from build123d import *

# Parameters (mm, degrees)
SKETCH1_R           = 1.5
SKETCH1_R_2         = 4.925
SKETCH1_W           = 9.9
SKETCH1_H           = 6.4
SKETCH1_W_2         = 6.4
SKETCH1_H_2         = 9.4
BOSS_EXTRUDE1_DEPTH = 6.4
SKETCH2_R           = 1.5
SKETCH2_W           = 6.4
SKETCH2_H           = 9.9
CUT_EXTRUDE1_DEPTH  = 415.760486883


with BuildPart() as part:
    # Sketch1 → Boss-Extrude1 (new body)
    with BuildSketch(Plane(origin=(0, 0, 0), x_dir=(0, 0, -1), z_dir=(1, 0, 0))):
        Polygon((210.165001125, 41.275232149), (-37.634998875, 41.275232149), (-73.734998875, 5.175232149), (-73.734998875, -333.674767851), (-33.721689147, -333.674767851), (-18.721689147, -318.674767851), (175.325001125, -318.674767851), (190.325001125, -333.674767851), (246.265001125, -333.674767851), (246.265001125, 5.175232149), align=None)
        with Locations((6.365001125, 34.475232149)):
            Circle(SKETCH1_R, mode=Mode.SUBTRACT)
        with Locations((86.365001125, 34.475232149)):
            Circle(SKETCH1_R, mode=Mode.SUBTRACT)
        with Locations((166.365001125, 34.475232149)):
            Circle(SKETCH1_R, mode=Mode.SUBTRACT)
        with Locations((86.46500109, -259.124767851)):
            Circle(SKETCH1_R, mode=Mode.SUBTRACT)
        with Locations((166.465001125, -259.124767851)):
            Circle(SKETCH1_R, mode=Mode.SUBTRACT)
        with Locations((6.46500109, -259.124767851)):
            Circle(SKETCH1_R, mode=Mode.SUBTRACT)
        with Locations((239.465001125, -29.824767851)):
            Circle(SKETCH1_R, mode=Mode.SUBTRACT)
        with Locations((239.465001125, -136.224767851)):
            Circle(SKETCH1_R, mode=Mode.SUBTRACT)
        with Locations((239.465001125, -242.624767851)):
            Circle(SKETCH1_R, mode=Mode.SUBTRACT)
        with Locations((-66.934998875, -242.624767851)):
            Circle(SKETCH1_R, mode=Mode.SUBTRACT)
        with Locations((-66.934998875, -136.224767851)):
            Circle(SKETCH1_R, mode=Mode.SUBTRACT)
        with Locations((-66.934998875, -29.824767851)):
            Circle(SKETCH1_R, mode=Mode.SUBTRACT)
        with Locations((224.265001125, 13.800232149)):
            Circle(SKETCH1_R_2, mode=Mode.SUBTRACT)
        with Locations((-51.734998875, 13.800232149)):
            Circle(SKETCH1_R_2, mode=Mode.SUBTRACT)
        with Locations((193.115001125, -15.324767851)):
            Circle(SKETCH1_R, mode=Mode.SUBTRACT)
        with Locations((193.115001125, -34.074767851)):
            Circle(SKETCH1_R, mode=Mode.SUBTRACT)
        with Locations((151.365001054, 34.475232149)):
            Rectangle(SKETCH1_W, SKETCH1_H, mode=Mode.SUBTRACT)
        with Locations((181.365001197, 34.475232149)):
            Rectangle(SKETCH1_W, SKETCH1_H, mode=Mode.SUBTRACT)
        with Locations((71.365001054, 34.475232149)):
            Rectangle(SKETCH1_W, SKETCH1_H, mode=Mode.SUBTRACT)
        with Locations((101.365001197, 34.475232149)):
            Rectangle(SKETCH1_W, SKETCH1_H, mode=Mode.SUBTRACT)
        with Locations((21.465001197, -259.124767851)):
            Rectangle(SKETCH1_W, SKETCH1_H, mode=Mode.SUBTRACT)
        Polygon((157.825001125, 6.525232149), (189.675001125, -25.324767851), (189.675001125, -206.824767851), (-34.371689147, -206.824767851), (-34.371689147, -25.324767851), (-2.521689147, 6.525232149), align=None, mode=Mode.SUBTRACT)
        Polygon((-3.584998946, -255.924767851), (-3.584999089, -262.324767851), (-13.484999089, -262.324767851), (-13.484998946, -255.924767851), align=None, mode=Mode.SUBTRACT)
        with Locations((101.465001197, -259.124767851)):
            Rectangle(SKETCH1_W, SKETCH1_H, mode=Mode.SUBTRACT)
        with Locations((-8.634998946, 34.475232149)):
            Rectangle(SKETCH1_W, SKETCH1_H, mode=Mode.SUBTRACT)
        with Locations((21.365001197, 34.475232149)):
            Rectangle(SKETCH1_W, SKETCH1_H, mode=Mode.SUBTRACT)
        Polygon((76.415001054, -255.924767851), (76.415000911, -262.324767851), (66.515000911, -262.324767851), (66.515001054, -255.924767851), align=None, mode=Mode.SUBTRACT)
        with Locations((239.465001125, -44.824767851)):
            Rectangle(SKETCH1_W_2, SKETCH1_H_2, mode=Mode.SUBTRACT)
        with Locations((151.465001125, -259.124767851)):
            Rectangle(SKETCH1_W, SKETCH1_H, mode=Mode.SUBTRACT)
        with Locations((181.465001125, -259.124767851)):
            Rectangle(SKETCH1_W, SKETCH1_H, mode=Mode.SUBTRACT)
    extrude(amount=BOSS_EXTRUDE1_DEPTH)

    # Sketch2 → Cut-Extrude1 (cut, through all)
    with BuildSketch(Plane(origin=(6.4, 0, 0), x_dir=(0, 0, -1), z_dir=(1, 0, 0))):
        with Locations((-66.934998875, -242.624767851)):
            Circle(SKETCH2_R)
        with Locations((-66.934998875, -136.224767851)):
            Circle(SKETCH2_R)
        with Locations((-66.934998875, -29.824767851)):
            Circle(SKETCH2_R)
        with Locations((239.465001125, -136.224767851)):
            Circle(SKETCH2_R)
        with Locations((239.465001125, -242.624767851)):
            Circle(SKETCH2_R)
        with Locations((239.465001125, -29.824767851)):
            Circle(SKETCH2_R)
        with Locations((-66.934998875, -257.624767851)):
            Rectangle(SKETCH2_W, SKETCH2_H)
        with Locations((-66.934998875, -227.624767851)):
            Rectangle(SKETCH2_W, SKETCH2_H)
        with Locations((-66.934998875, -121.224767851)):
            Rectangle(SKETCH2_W, SKETCH2_H)
        with Locations((-66.934998875, -151.224767851)):
            Rectangle(SKETCH2_W, SKETCH2_H)
        with Locations((-66.934998875, -14.824767851)):
            Rectangle(SKETCH2_W, SKETCH2_H)
        with Locations((-66.934998875, -44.824767851)):
            Rectangle(SKETCH2_W, SKETCH2_H)
        with Locations((239.465001125, -121.224767851)):
            Rectangle(SKETCH2_W, SKETCH2_H)
        with Locations((239.465001125, -151.224767851)):
            Rectangle(SKETCH2_W, SKETCH2_H)
        with Locations((239.465001125, -227.624767851)):
            Rectangle(SKETCH2_W, SKETCH2_H)
        with Locations((239.465001125, -257.624767851)):
            Rectangle(SKETCH2_W, SKETCH2_H)
        with Locations((239.465001125, -14.824767851)):
            Rectangle(SKETCH2_W, SKETCH2_H)
        with Locations((239.465001125, -44.824767851)):
            Rectangle(SKETCH2_W, SKETCH2_H)
    extrude(amount=-CUT_EXTRUDE1_DEPTH, mode=Mode.SUBTRACT)


solid = part.part
Could you check a few things on this model? Use its own coordinates, in mm. A direction names the side the tool comes from. Give positions to 0.01 mm unless a question says otherwise; leave off trailing zeros. Order: outer loops, then holes, each group sorted by start corner. A loop starts at its lowest first (then second) coordinate and runs counter-clockwise, first axis right, second up.
Item 1: If we section it at D-D, the plane x = 3.25: Count the separate pieces of the cut face and the enclosed holes in it, plus the area to 3 significant figures.
Item 2: If we mould it in two halves opening along Z, with no side actions, what happens to faces 1 (the face through (6.4, -227, -84)), 2 (the face through (3.155, -9.623, 18.67)), 3 (the face through (3.16, 23.48, 55.43))? For each: pulls with the +Z half, pulls with the -Z half, needs draft (parallel to the pull), parting line crosses it, or undercut.
Item 3: If we section it at C-C, the plane z = -57: Write out the boundary of the cut face in (x, y).
Item 4: For faces 4 (the face through (3.155, -326.28, 26.327)), 5 (the face through (3.16, -9.18, -173.53)), 6 (the face through (0, -227, -84)), which set-ups out of +Z, -Z, +X, -X, +Y, -Y let a thin tool reach every point of the face, with its end or its side?
Item 5: I need wall thicknesses on line 1 (Z direction, x = 5.5, y = -149.5) (3 decimals); line 2 (Y direction, x = 2.25, z = -19.5); line 3 (Y direction, x = 4, z = -29). Which ranges of each line are inside material? Lowest first, please.
Item 6: I'm going to push flat-ended pins straight in: pin 1 (2.5 mm diameter, centred on y = -34.07, z = -193.12, fed in from -X); pin 2 (1 mm diameter, centred on x = 5.5, z = 1, fed in from -Y); pin 3 (1.9 mm diameter, centred on x = 4.5, y = 35, fed in from +Z); pin 4 (1.5 mm diameter, centred on y = -136, z = -204.5, fed in from -X). Where does each tip first touch, or does it pass through?
Item 7: If we section it at A-A, the plane y = -86.5: Write out the boundary of the cut face in (x, z) (3 decimals).
Item 8: If we section it at B-B, the plane z = -152: Write out the boundary of the cut face in (x, y).
Values:
1. separate pieces: 1
1. enclosed holes: 41
1. area: 67,000 mm2
2. face 1: needs draft
2. face 2: undercut
2. face 3: pulls with the +Z half
3. outline: (0, -318.67) - (6.4, -318.67) - (6.4, -206.82) - (0, -206.82) - close; (0, 6.53) - (6.4, 6.53) - (6.4, 41.28) - (0, 41.28) - close
4. face 4: +X, -X, -Y
4. face 5: +X, -X
4. face 6: +Z, -Z, -X, +Y, -Y
5. line 1: z = -246.265 to -242.665, -236.265 to -189.675, 34.372 to 63.735, 70.135 to 73.735
5. line 2: y = -318.67 to -262.32, -255.92 to -206.82, 6.53 to 31.28, 37.68 to 41.28
5. line 3: y = -318.67 to -206.82, 6.53 to 41.28
6. pin 1: passes through
6. pin 2: stops at y = -318.67
6. pin 3: stops at z = 44.86
6. pin 4: stops at x = 0
7. outline: (0, -246.265) - (6.4, -246.265) - (6.4, -189.675) - (0, -189.675) - close; (0, 34.372) - (6.4, 34.372) - (6.4, 73.735) - (0, 73.735) - close
8. outline: (0, -318.67) - (6.4, -318.67) - (6.4, -262.32) - (0, -262.32) - close; (0, -255.92) - (6.4, -255.92) - (6.4, -206.82) - (0, -206.82) - close; (0, 6.53) - (6.4, 6.53) - (6.4, 31.28) - (0, 31.28) - close; (0, 37.68) - (6.4, 37.68) - (6.4, 41.28) - (0, 41.28) - close
